Read the model definition and answer for the solid it produces. Units are mm, in the model's axes. A direction names the side the tool comes from. Round coordinates to 2 decimals unless told otherwise and drop trailing zeros. Write each loop counter-clockwise with the first axis right and the second up, starting at its lowest first coordinate (ties: lowest second). Pieces come first, ordered by that corner, then holes. Notation, with made-up numbers: (7, 83.25) -> (54, 83.25) arc R25 ccw to (54, 101.25) -> close; hole circle Ø8 at (52.25, 16). An arc over 180 degrees is marked (long way). Return JSON: item names as keys, results as strings. Group by question number.
(1) A cutting plane is placed at C-C on y = 1.5. Give the vertices of the cut face in (x, z).
(2) A cutting plane is placed at A-A on z = 1.25. Give the vertices of the cut face in (x, y).
(3) For faces 1 (the flat face through (8.957, 9, 3)), 2 (the flat face through (9.009, 0, 3)), 3 (the flat face through (-9.009, 0, 3)), 4 (the cylindrical face through (0, -4.5, 3.5)), determine the directions among +Z, -Z, +X, -X, +Y, -Y from which every point of the face is accessible in a straight line to the end or side of a thin tool.
(4) A cutting plane is placed at B-B on x = 7. Give the vertices of the cut face in (y, z), then the cut area to 3 significant figures.
(5) A cutting plane is placed at D-D on x = 2. Give the vertices of the cut face in (y, z), then the cut area to 3 significant figures.
(6) Given pin 1 (2 mm diameter, centred on x = 1.5, z = 5.5, fed in from +Y); pin 2 (4 mm diameter, centred on x = -12.5, y = 8.5, fed in from +Z); pin 3 (3 mm diameter, centred on y = 9, z = 5, fed in from -X); pin 4 (6 mm diameter, centred on x = 0.5, y = 22, fed in from +Z), each flat-ended and moving along its own axis, determine where each tip first touches the part or whether it passes through.
(7) Straight lines are drawn through the part: line 1 (Z direction, x = -3, y = 34.5); line 2 (Y direction, x = 4.5, z = 4); line 3 (X direction, y = 8, z = 5). For each, find the intervals that lie inside material, in ascending order.
(8) The mould has two halves that part along X. Classify faces 5 (the flat face through (-8.957, 9, 3)), 6 (the flat face through (24, 26, 1)), 7 (the cylindrical face through (0, 4.5, 3.5)): released by +X, released by -X, zero draft, split by the parting line, or undercut.
```python
from build123d import *

# Parameters (mm, degrees)
F1_DEPTH = 7
F2_DEPTH = 3
F3_W     = 48
F3_H     = 3
F4_DEPTH = 27


with BuildPart() as f1:
    # F0 (on Top) → F1 (new body)
    with BuildSketch(Plane.XY):
        Polygon((0.000171, 8.035728), (-6.356564, 8.035728), (-8.956735, 8.035728), (-9.009132, 8.035728), (-9.009132, -7.608017), (9.009474, -7.608017), (9.009474, 8.035728), (8.956735, 8.035728), (6.356564, 8.035728), align=None)
        with BuildLine():
            Line((3.00302, 3.351398), (2.996931, -3.356845))
            ThreePointArc((2.996931, -3.356845), (-0.004116, -4.499998), (-3.003067, -3.351357))
            Line((-3.003067, -3.351357), (-2.996977, 3.356803))
            ThreePointArc((-2.996977, 3.356803), (0.004054, 4.499998), (3.00302, 3.351398))
        make_face(mode=Mode.SUBTRACT)
        Polygon((-8.956735, 8.035728), (-6.356564, 8.035728), (0.000171, 8.035728), (6.356564, 8.035728), (8.956735, 8.035728), (8.956735, 10.535728), (0, 10.535728), (-8.956735, 10.535728), align=None)
    extrude(amount=F1_DEPTH)

    # F0 (on Top) → F2 (join)
    with BuildSketch(Plane.XY):
        Polygon((-24, 10.535728), (-8.956735, 10.535728), (0, 10.535728), (8.956735, 10.535728), (24, 10.535728), (24, 15.535728), (0, 15.535728), (-24, 15.535728), align=None)
    extrude(amount=F2_DEPTH)

    # F3 (on face) → F4 (join)
    with BuildSketch(Plane(origin=(0, 15.535728, 0), x_dir=(-1, 0, 0), z_dir=(0, 1, 0))):
        with Locations((0, 1.5)):
            Rectangle(F3_W, F3_H)
    extrude(amount=F4_DEPTH)


solid = f1.part
```
Checks:
{
 "1": {"outline": "(-9.01, 0) -> (-3, 0) -> (-3, 7) -> (-9.01, 7) -> close; (3, 0) -> (9.01, 0) -> (9.01, 7) -> (3, 7) -> close"},
 "2": {"outline": "(-24, 10.54) -> (-8.96, 10.54) -> (-8.96, 8.04) -> (-9.01, 8.04) -> (-9.01, -7.61) -> (9.01, -7.61) -> (9.01, 8.04) -> (8.96, 8.04) -> (8.96, 10.54) -> (24, 10.54) -> (24, 42.54) -> (-24, 42.54) -> close; hole (-3, -3.35) arc R4.5 ccw to (3, -3.36) -> (3, 3.35) arc R4.5 ccw to (-3, 3.36) -> close"},
 "3": {"face 1": "+Z, -Z, +X", "face 2": "+Z, -Z, +X, -Y", "face 3": "+Z, -Z, -X, -Y", "face 4": "+Z, -Z"},
 "4": {"outline": "(-7.61, 0) -> (42.54, 0) -> (42.54, 3) -> (10.54, 3) -> (10.54, 7) -> (-7.61, 7) -> close", "area": "223 mm^2"},
 "5": {"outline": "(-7.61, 0) -> (-4.03, 0) -> (-4.03, 7) -> (-7.61, 7) -> close; (4.03, 0) -> (42.54, 0) -> (42.54, 3) -> (10.54, 3) -> (10.54, 7) -> (4.03, 7) -> close", "area": "167 mm^2"},
 "6": {"pin 1": "stops at y = 10.54", "pin 2": "passes through", "pin 3": "stops at x = -9.01", "pin 4": "stops at z = 3"},
 "7": {"line 1": "z = 0 to 3", "line 2": "y = -7.61 to 10.54", "line 3": "x = -9.01 to 9.01"},
 "8": {"face 5": "released by -X", "face 6": "released by +X", "face 7": "undercut"}
}
